Part print with two shaded views. Sizes in mm from the minimum x, y, z corner. A direction names the side the tool comes from. Round coordinates to 2 decimals unless told otherwise and drop trailing zeros. Write each loop counter-clockwise with the first axis right and the second up, starting at its lowest first coordinate (ties: lowest second). Pieces come first, ordered by that corner, then holes. Notation, with made-up numbers: (17, -19) -> (73, -19) arc R34 ccw to (73, 20) -> close; hole circle Ø1 at (12, 55.25). An arc over 180 degrees is marked (long way). Return JSON: item names as keys, results as strings.
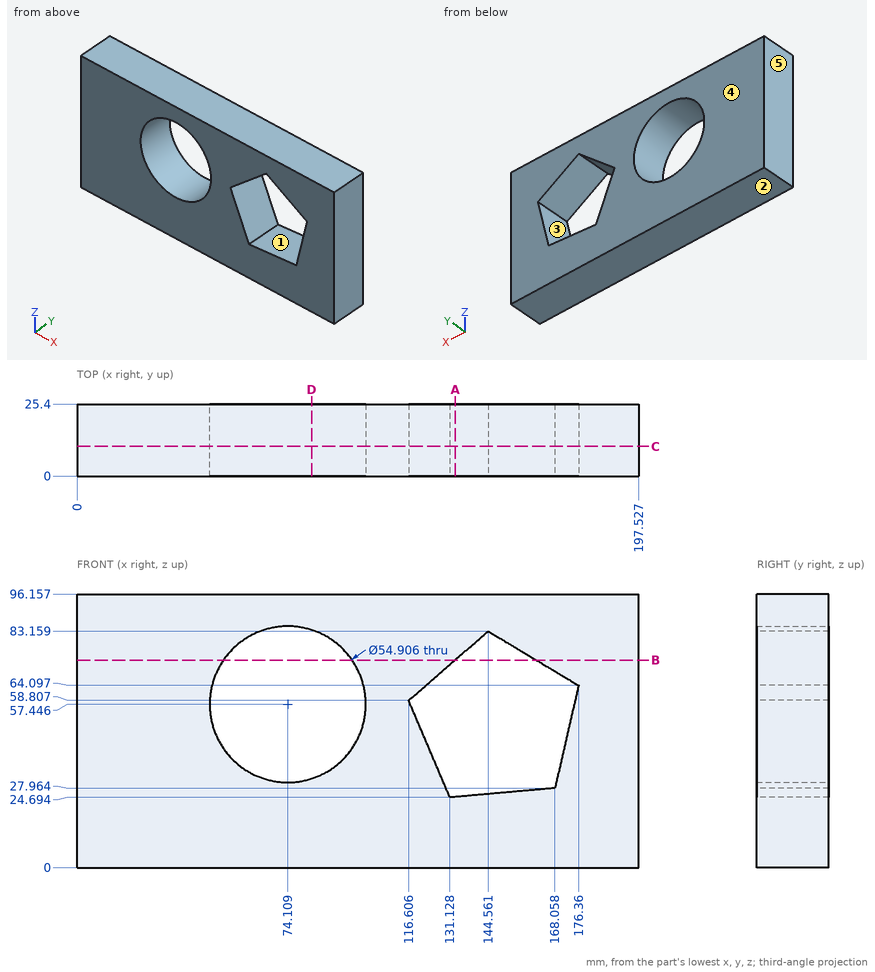
Q1. Wall check: L1, parallel to X at y = 5.25, z = 51.5 (1 decimal); L2, parallel to X at y = 20.25, z = 75 (1 decimal); L3, parallel to Z at x = 52, y = 19.75 (1 decimal). Give the ranges that are in metal, low to high.
Verdict:
{"L1": "x = 0 to 47.3, 100.9 to 119.7, 173.5 to 197.5", "L2": "x = 0 to 53, 95.2 to 135.2, 158.2 to 197.5", "L3": "z = 0 to 41.2, 73.7 to 96.2"}
Q2. Two-plate mould, pull along X, no slides. Class the marked faces 3, 4 and 5: +X half, -X half, draft (parallel to the pull), parting line (faces both ways), or undercut.
Verdict:
{"face 3": "undercut", "face 4": "draft", "face 5": "-X half"}
Q3. Saw through at C-C on y = 10.5. List the corners of the cut face in (x, z) (1 decimal).
Verdict:
{"outline": "(0, 0) -> (197.5, 0) -> (197.5, 96.2) -> (0, 96.2) -> close; hole circle Ø54.9 at (74.1, 57.4); hole (116.6, 58.8) -> (131.1, 24.7) -> (168.1, 28) -> (176.4, 64.1) -> (144.6, 83.2) -> close"}
Q4. 3-axis set-ups, long thin cutter, end or side, ignore diameter. For the marked faces 1 and 2: which of +Z, -Z, +X, -X, +Y, -Y reach the whole face in a straight line?
Verdict:
{"face 1": "+Y, -Y", "face 2": "-Z, +X, -X, +Y, -Y"}
Q5. Saw through at B-B on z = 73. List the corners of the cut face in (x, y), then the cut area to 3 significant figures.
Verdict:
{"outline": "(0, 0) -> (51.49, 0) -> (51.49, 25.4) -> (0, 25.4) -> close; (96.73, 0) -> (132.9, 0) -> (132.9, 25.4) -> (96.73, 25.4) -> close; (161.51, 0) -> (197.53, 0) -> (197.53, 25.4) -> (161.51, 25.4) -> close", "area": "3,140 mm²"}
Q6. Saw through at D-D on x = 82.5. List the corners of the cut face in (y, z) (1 decimal).
Verdict:
{"outline": "(0, 0) -> (25.4, 0) -> (25.4, 31.3) -> (0, 31.3) -> close; (0, 83.6) -> (25.4, 83.6) -> (25.4, 96.2) -> (0, 96.2) -> close"}
Q7. Saw through at A-A on x = 133. List the corners of the cut face in (y, z), then the cut area to 3 significant figures.
Verdict:
{"outline": "(0, 0) -> (25.4, 0) -> (25.4, 24.86) -> (0, 24.86) -> close; (0, 73.09) -> (25.4, 73.09) -> (25.4, 96.16) -> (0, 96.16) -> close", "area": "1,220 mm²"}
